Autodesk Inventor part; units mm, degrees
ref_plane "YZ Plane" through (0, 0, 0) normal (1, 0, 0) x (0, 1, 0)
ref_plane "XZ Plane" through (0, 0, 0) normal (0, 1, 0) x (-1, 0, 0)
ref_plane "XY Plane" through (0, 0, 0) normal (0, 0, 1) x (1, 0, 0)
sketch "Sketch1" plane through (0, 0, 0) normal (0, 0, 1) x (1, 0, 0)
  line L0 (-6.35, -3.6662) -> (-6.35, 3.6662)
  line L1 (-6.35, 3.6662) -> (0, 7.3323)
  line L2 (0, 7.3323) -> (6.35, 3.6662)
  line L3 (6.35, 3.6662) -> (6.35, -3.6662)
  line L4 (6.35, -3.6662) -> (0, -7.3323)
  line L5 (0, -7.3323) -> (-6.35, -3.6662)
  point P0 (0, 0)
  point P1 (0, 0)
  dimension "Size" = 12.7
extrude "Extrusion1" add sketch "Sketch1" along normal mid plane 127
sketch "Sketch3" plane through (0, 0, 63.5) normal (0, 0, 1) x (1, 0, 0)
  line L0 (-6.35, 3.6662) -> (0, 7.3323) construction
  line L1 (0, 7.3323) -> (6.35, 3.6662) construction
  line L2 (6.35, 3.6662) -> (6.35, -3.6662) construction
  line L3 (6.35, -3.6662) -> (0, -7.3323) construction
  line L4 (0, -7.3323) -> (-6.35, -3.6662) construction
  line L5 (-6.35, -3.6662) -> (-6.35, 3.6662) construction
  point P0 (0, 0)
hole "Hole1" at (0, 0, 63.5) direction (0, 0, -1) diameter 5.1054 end through all
sketch "Sketch4" plane through (0, 0, 63.5) normal (0, 0, 1) x (1, 0, 0)
  circle A0 centre (0, 0) radius 2.5527 construction
  line L0 (-6.35, 3.6662) -> (0, 7.3323) construction
  line L1 (0, 7.3323) -> (6.35, 3.6662) construction
  line L2 (6.35, 3.6662) -> (6.35, -3.6662) construction
  line L3 (6.35, -3.6662) -> (0, -7.3323) construction
  line L4 (0, -7.3323) -> (-6.35, -3.6662) construction
  line L5 (-6.35, -3.6662) -> (-6.35, 3.6662) construction
  circle A1 centre (0, 0) radius 6.8771
  circle A2 centre (0, 0) radius 8.89
  dimension "thunder" = 13.7541
  dimension "d16" = 17.78
extrude "Extrusion3" cut sketch "Sketch4" against normal through all
sketch "Sketch5" plane through (0, 0, 63.5) normal (0, 0, 1) x (1, 0, 0)
  arc A0 (5.4616, -4.1791) -> (6.35, -2.6403) centre (0, 0) ccw
  line L0 (6.35, -2.6403) -> (6.35, 2.6403)
  arc A1 (6.35, 2.6403) -> (5.4616, 4.1791) centre (0, 0) ccw
  line L1 (5.4616, 4.1791) -> (0.8884, 6.8194)
  arc A2 (0.8884, 6.8194) -> (-0.8884, 6.8194) centre (0, 0) ccw
  line L2 (-0.8884, 6.8194) -> (-5.4616, 4.1791)
  arc A3 (-5.4616, 4.1791) -> (-6.35, 2.6403) centre (0, 0) ccw
  line L3 (-6.35, 2.6403) -> (-6.35, -2.6403)
  arc A4 (-6.35, -2.6403) -> (-5.4616, -4.1791) centre (0, 0) ccw
  line L4 (-5.4616, -4.1791) -> (-0.8884, -6.8194)
  arc A5 (-0.8884, -6.8194) -> (0.8884, -6.8194) centre (0, 0) ccw
  line L5 (0.8884, -6.8194) -> (5.4616, -4.1791)
  circle A6 centre (0, 0) radius 2.5527
  circle A7 centre (0, 0) radius 6.35
  point P0 (3.175, -5.4993)
  point P1 (-3.175, -5.4993)
  point P2 (-6.35, 0)
  point P3 (-3.175, 5.4993)
  point P4 (3.175, 5.4993)
  point P5 (6.35, 0)
  dimension "d19" = 12.7
extrude "Extrusion4" cut sketch "Sketch5" against normal blind 8.001 contours L5 A7 L0 A0 | L5 A5 L4 A7 | A7 L1 A1 L0 | L4 A4 L3 A7 | A7 L2 A2 L1 | L3 A3 L2 A7
mirror "Mirror2" about plane through (0, 0, 0) normal (0, 0, 1) of "Extrusion4"
equation "\"bearing\" = 25.4"
properties part number "GP3-002" material "Aluminum 6061"
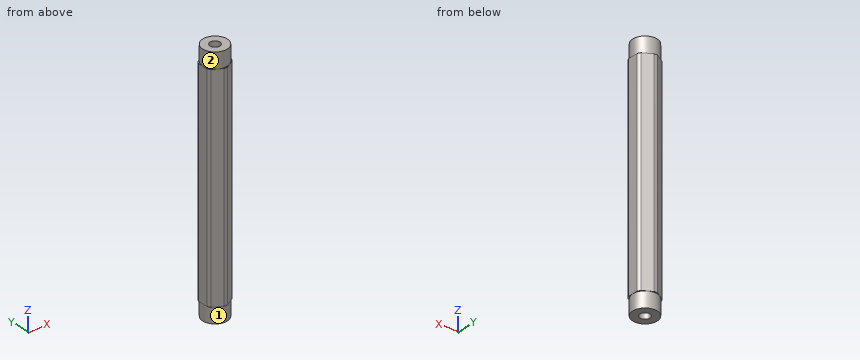
Geometry: final body of the model. Coordinates: model frame, mm. Face numbers are marked on the shaded views. A direction names the side the tool comes from. Coordinates: 2 decimals unless noted, no trailing zeros. Write each loop counter-clockwise with the first axis right and the second up, starting at its lowest first coordinate (ties: lowest second). Pieces come first, ordered by that corner, then holes. Notation, with made-up numbers: (-37.5, 42) - (-12.5, 42) arc R11 ccw to (-12.5, 46) - close; hole circle Ø6 at (65.5, -35.75). An arc over 180 degrees is marked (long way). Return JSON: item names as keys, results as strings.
Item 1: Reachability of the marked faces 1 and 2 from +Z, -Z, +X, -X, +Y, -Y: full face, straight path, thin tool, end or side. Return the list, or none.
Completed:
{"face 1": "-Z", "face 2": "+Z"}
Item 2: Pin query (flat end, axial travel): pin 1 Ø0.7 at (x, y) = (1, 6.5) entering from -Z. Return the tip coordinate at first contact, or that it passes through.
Completed:
{"pin 1": "stops at z = -63.5"}
Item 3: Section query A-A (y = 1.25). Output: boundary loops of the cut face in (x, z), and give its area (3 significant figures).
Completed:
{"outline": "(-6.35, -55.5) - (-6.23, -55.5) - (-6.23, -63.5) - (-2.23, -63.5) - (-2.23, 63.5) - (-6.23, 63.5) - (-6.23, 55.5) - (-6.35, 55.5) - close; (2.23, -63.5) - (6.23, -63.5) - (6.23, -55.5) - (6.35, -55.5) - (6.35, 55.5) - (6.23, 55.5) - (6.23, 63.5) - (2.23, 63.5) - close", "area": "1,040 mm2"}
Item 4: Section query B-B (z = 5). Output: boundary loops of the cut face in (x, y).
Completed:
{"outline": "(-6.35, -2.64) arc R6.88 ccw to (-5.46, -4.18) - (-0.89, -6.82) arc R6.88 ccw to (0.89, -6.82) - (5.46, -4.18) arc R6.88 ccw to (6.35, -2.64) - (6.35, 2.64) arc R6.88 ccw to (5.46, 4.18) - (0.89, 6.82) arc R6.88 ccw to (-0.89, 6.82) - (-5.46, 4.18) arc R6.88 ccw to (-6.35, 2.64) - close; hole circle Ø5.11 at (0, 0)"}
Item 5: Line query: L1, parallel to X at y = 0, z = -17.5; L2, parallel to Y at x = 0, z = -32.5; L3, parallel to X at y = 0.25, z = -34. Output: solid intervals per line, ascending.
Completed:
{"L1": "x = -6.35 to -2.55, 2.55 to 6.35", "L2": "y = -6.88 to -2.55, 2.55 to 6.88", "L3": "x = -6.35 to -2.54, 2.54 to 6.35"}
